Geometry: final body of the model. Coordinates: model frame, mm. Face numbers are marked on the shaded views. A direction names the side the tool comes from. Give positions to 0.01 mm unless a question says otherwise; leave off trailing zeros. Order: outer loops, then holes, each group sorted by start corner. A loop starts at its lowest first (then second) coordinate and runs counter-clockwise, first axis right, second up. Notation, with made-up numbers: M -31,-37.5 L 8,-37.5 A25 ccw 8,-21.5 Z; hole C -14.5,-15.75 d6. An arc over 180 degrees is marked long. Write item = value, one per line. Start each with the question number.
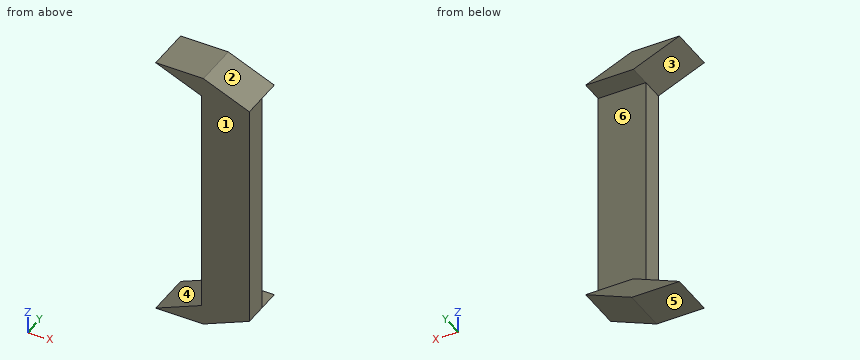
from build123d import *

# Parameters (mm, degrees)
SKETCH1_W           = 6.4
SKETCH1_H           = 30.61
BOSS_EXTRUDE1_DEPTH = 3
BOSS_EXTRUDE2_DEPTH = 6


with BuildPart() as part:
    # Sketch1 → Boss-Extrude1 (new body)
    with BuildSketch(Plane(origin=(0, 0, 0), x_dir=(1, 0, 0), z_dir=(0, 1, 0))):
        Rectangle(SKETCH1_W, SKETCH1_H)
    extrude(amount=BOSS_EXTRUDE1_DEPTH)

    # Sketch1_3 → Boss-Extrude2 (add)
    with BuildSketch(Plane(origin=(0, 0, 0), x_dir=(1, 0, 0), z_dir=(0, 1, 0))):
        Polygon((3.2, -15.305), (-2.966154938, -17.922377484), (-9.366154938, -17.922377484), (-3.2, -15.305), align=None)
        Polygon((3.2, 15.305), (-2.966154938, 17.922377484), (-9.366154938, 17.922377484), (-3.2, 15.305), align=None)
    extrude(amount=BOSS_EXTRUDE2_DEPTH)


solid = part.part
1) Access query for the marked faces 4, 5 and 6. Directions: +Z, -Z, +X, -X, +Y, -Y. A direction counts if a zero-diameter tool reaches every point of the face in a straight line with its end or side. Return the directions, or none.
2) Cut plane C-C (y = 1.4). Return loops of the section in (x, z) (3 decimals), plus the area to 3 significant figures.
3) Pin query (flat end, axial travel): pin 1 Ø5 at (x, z) = (1, 6) entering from +Y; pin 2 Ø3 at (x, y) = (2, 4) entering from -Z; pin 3 Ø0.9 at (x, y) = (-1, 4) entering from +Z. Return the tip coordinate at first contact, or that it passes through.
4) Cut plane B-B (x = -6). Return loops of the section in (y, z), plus the area to 3 significant figures.
5) Cut plane A-A (y = 5.05). Return loops of the section in (x, z) (3 decimals), plus the area to 3 significant figures.
6) Draft query along Z for the marked faces 1, 2 and 3. Return one class per face: pulls with the +Z half, pulls with the -Z half, needs draft (parallel to the pull), parting line crosses it, or undercut.
7) Ray query, L1, parallel to X at y = 2.6, z = 2; L2, parallel to Y at x = -1.5, z = -6.5; L3, parallel to Z at x = 0, y = 3.15 (3 decimals). Return the intervals inside material, ascending.
8) Cut plane D-D (z = 10.5). Return loops of the section in (x, y).
Reply:
q1.face_4 = -X, +Y, -Y
q1.face_5 = -Z, +X, -X, +Y, -Y
q1.face_6 = +X, -X, +Y
q2.outline = M -9.366,-17.922 L -2.966,-17.922 L 3.2,-15.305 L 3.2,15.305 L -2.966,17.922 L -9.366,17.922 L -3.2,15.305 L -3.2,-15.305 Z
q2.area = 229 mm²
q3.pin_1 = 3
q3.pin_2 = -16.45
q3.pin_3 = 17.28
q4.outline = M 0,-17.92 L 6,-17.92 L 6,-16.49 L 0,-16.49 Z; M 0,16.49 L 6,16.49 L 6,17.92 L 0,17.92 Z
q4.area = 17.1 mm²
q5.outline = M -9.366,-17.922 L -2.966,-17.922 L 3.2,-15.305 L -3.2,-15.305 Z; M -9.366,17.922 L -3.2,15.305 L 3.2,15.305 L -2.966,17.922 Z
q5.area = 33.5 mm²
q6.face_1 = needs draft
q6.face_2 = pulls with the +Z half
q6.face_3 = undercut
q7.L1 = -3.2 to 3.2
q7.L2 = 0 to 3
q7.L3 = -16.663 to -15.305, 15.305 to 16.663
q8.outline = M -3.2,0 L 3.2,0 L 3.2,3 L -3.2,3 Z
